Model file for the job. Use its own axes, mm. A direction names the side the tool comes from. Round coordinates to 2 decimals unless told otherwise and drop trailing zeros. Write item = value, one per line.
```python
from build123d import *

# Parameters (mm, degrees)
BOSS_EXTRUDE1_OUTLINE_R   = 1.411527177
BOSS_EXTRUDE1_OUTLINE_R_2 = 1.243983369
BOSS_EXTRUDE1_DEPTH       = 8.89
CUT_EXTRUDE1_START        = -4.445
SKETCH3_R                 = 2.54
CUT_EXTRUDE1_DEPTH        = 4.445
FILLET2_R                 = 3.556
SKETCH4_W                 = 38.788702954
SKETCH4_H                 = 29.49823266
CUT_EXTRUDE2_DEPTH        = 2.54
SKETCH5_R                 = 3.96875
CUT_EXTRUDE6_DEPTH        = 2.54
CUT_EXTRUDE9_DEPTH        = 4.445
CUT_EXTRUDE10_DEPTH       = 8.89


# Read off the part's stored shape, not the designer's step: Boss-Extrude1
with BuildPart() as part:
    # Boss-Extrude1 outline → Boss-Extrude1 (new body)
    with BuildSketch(Plane.XY):
        with BuildLine():
            add(Edge.make_bspline(
                [(-4.450270059, 36.453127637), (9.257211294, 37.68062732), (17.994865779, 35.108973576), (21.762693397, 28.738166405)],
                knots=[0.06260201, 0.06260201, 0.06260201, 0.06260201, 0.571198862, 0.571198862, 0.571198862, 0.571198862], degree=3))
            ThreePointArc((-4.450270059, 36.453127637), (-14.614683226, 26.381475664), (-1.480390785, 20.703110531))
            add(Edge.make_bspline(
                [(19.455202419, 25.136523629), (8.814175151, 23.55437226), (-1.480390785, 20.703110531)],
                knots=[0, 0, 0, 0.700849117, 0.700849117, 0.700849117], degree=2))
            ThreePointArc((19.455202419, 25.136523629), (21.593913789, 26.306299678), (21.762693397, 28.738166405))
        make_face()
        with Locations((-6.128238366, 27.981709907)):
            Circle(BOSS_EXTRUDE1_OUTLINE_R, mode=Mode.SUBTRACT)
        with Locations((19.455202419, 27.676523629)):
            Circle(BOSS_EXTRUDE1_OUTLINE_R_2, mode=Mode.SUBTRACT)
    extrude(amount=BOSS_EXTRUDE1_DEPTH)

    # Sketch3 → Cut-Extrude1 (cut)
    with BuildSketch(Plane.XY.offset(8.89).offset(CUT_EXTRUDE1_START)):
        with Locations((19.455202419, 27.676523629)):
            Circle(SKETCH3_R)
    extrude(amount=CUT_EXTRUDE1_DEPTH, mode=Mode.SUBTRACT)

    # Fillet2
    fillet2_edges = [part.edges().sort_by_distance(p)[0] for p in [
        (-14.614683226, 26.381475664, 8.89),
        (8.919366654, 23.241027384, 8.89),
        (9.568834416, 36.110759147, 8.89),
    ]]
    fillet(fillet2_edges, radius=FILLET2_R)

    # Sketch4 → Cut-Extrude2 (cut)
    with BuildSketch(Plane(origin=(0, 0, 0), x_dir=(-1, 0, 0), z_dir=(0, 0, -1))):
        with Locations((-4.403454377, 29.061669641)):
            Rectangle(SKETCH4_W, SKETCH4_H)
    extrude(amount=-CUT_EXTRUDE2_DEPTH, mode=Mode.SUBTRACT)

    # Sketch5 → Cut-Extrude6 (cut)
    with BuildSketch(Plane.XY.offset(8.89)):
        with Locations((-6.128238366, 27.981709907)):
            Circle(SKETCH5_R)
    extrude(amount=-CUT_EXTRUDE6_DEPTH, mode=Mode.SUBTRACT)

    # Sketch11 → Cut-Extrude9 (cut)
    with BuildSketch(Plane.XY.offset(8.89)):
        Polygon((8.044294619, 22.027673787), (18.775840599, 28.536123817), (19.455202419, 27.676523629), (23.93696494, 27.676523629), (25.091261189, 21.861175279), (8.722262202, 18.612070842), align=None)
    extrude(amount=-CUT_EXTRUDE9_DEPTH, mode=Mode.SUBTRACT)

    # Sketch13 → Cut-Extrude10 (cut)
    with BuildSketch(Plane(origin=(0, 0, 2.54), x_dir=(-1, 0, 0), z_dir=(0, 0, -1))):
        with BuildLine():
            Line((10.206570894, 20.369371253), (8.596583203, 18.138185272))
            Line((8.596583203, 18.138185272), (1.153394416, 19.253778262))
            Line((1.153394416, 19.253778262), (1.535882515, 20.771294499))
            add(Edge.make_bspline(
                [(1.535882515, 20.771294499), (6.119525821, 19.09120268), (10.206570894, 20.369371253)],
                knots=[0, 0, 0, 0.81876004, 0.81876004, 0.81876004], degree=2))
        make_face()
    extrude(amount=-CUT_EXTRUDE10_DEPTH, mode=Mode.SUBTRACT)


solid = part.part
```
1) Flat gauge pins, fed straight in: pin 1 Ø1.5 at (y, z) = (34.5, 4.5) entering from +X; pin 2 Ø2 at (x, z) = (-10.5, 6) entering from +Y; pin 3 Ø3 at (x, y) = (19.46, 27.68) entering from +Z (3 decimals). Where does each tip first touch, or does it go through?
Conclusion:
pin_1 = 16.51
pin_2 = 35.89
pin_3 = 4.445
2) Wall check: line 1 along Z through (x, y) = (19, 29) (3 decimals); line 2 along Z through (x, y) = (-4, 33); line 3 along X through (y, z) = (30.5, 8.25). Give the ranges that are in metal, low to high.
Conclusion:
line_1 = 2.54 to 4.445
line_2 = 2.54 to 8.89
line_3 = -12.78 to -9.2, -3.06 to 18.42
3) 3-axis set-ups, long thin cutter, end or side, ignore diameter. For faces 1 (the face through (18, 27, 4.445)), 2 (the face through (3, 29, 8.89)), 3 (the face through (-6.989, 24.107, 7.638)): which of +Z, -Z, +X, -X, +Y, -Y reach the whole face in a straight line?
Conclusion:
face_1 = +Z, -Y
face_2 = +Z, +X, -X, +Y, -Y
face_3 = +Z
4) Mould opens along X. For faces 4 (the face through (0, 28, 2.54)), 5 (the face through (14.43, 25.9, 6.16)), 6 (the face through (19.29, 28.91, 3.48)) say: +X half, -X half, draft (parallel to the pull), parting line (faces both ways), or undercut.
Conclusion:
face_4 = draft
face_5 = +X half
face_6 = undercut
